Build history of the part. All positions in model axes, mm. A direction names the side the tool comes from. Give positions to 0.01 mm unless a question says otherwise; leave off trailing zeros. Loops run counter-clockwise (first coordinate to the right, second up) from the corner with the lowest first, then second, coordinate; pieces in that order, holes last. Notation, with made-up numbers: (-17, -27) -> (17, -27) arc R13 cw to (17, -4) -> close; hole circle Ø6 at (17, 84.25). An arc over 180 degrees is marked (long way). Answer as a JSON object with one key per item and string values. Group by question number.
Q1. Band-saw the part on C-C, the plane z = 1.5. Count the separate pieces of the cut face and the enclosed holes in it, plus the area to 3 significant figures.
Q2. Band-saw the part on A-A, the plane z = 11.25. Write the cut outline in (x, y).
Q3. Drop flat-ended pins along their axis: pin 1 (1.9 mm diameter, centred on x = 14.58, y = -9.94, fed in from +Z); pin 2 (2.5 mm diameter, centred on x = -15.5, y = 8, fed in from +Z); pin 3 (3.5 mm diameter, centred on x = -16.97, y = -16.97, fed in from -Z). Give the stop position or say it passes through.
Q4. Two-plate mould, pull along Y, no slides. Class faces 4 (the flat face through (15, 10, 2)), 5 (the cylindrical face through (19.797, -19.859, 7.605)), 6 (the flat face through (-21, 0, 7)): pulls with the +Y half, pulls with the -Y half, needs draft (parallel to the pull), parting line crosses it, or undercut.
Q5. Wall check: probe 1 along X at (y, z) = (-0.5, 4.25); probe 2 along X at (y, z) = (14.5, 3); probe 3 along X at (y, z) = (-5.5, 2.5). Give the ranges that are in metal, low to high. Write a range as from..to.
Q6. Band-saw the part on B-B, the plane y = 5. Write the cut outline in (x, z).
Q7. Tool access for faces 1 (the cylindrical face through (-19.02, -16.32, 2.96)), 2 (the flat face through (-4, -17, 2)), 3 (the flat face through (20, -1.1, 14)): list every direction of +Z, -Z, +X, -X, +Y, -Y with a clear straight run to the whole face (end or side of a thin tool).
from build123d import *

# Parameters (mm, degrees)
SKETCH_1_W               = 42
SKETCH_1_H               = 42
EXTRUDE_1_DEPTH          = 15
FILLET_2_R               = 4
SKETCH_25_R              = 1.15
CUT_EXTRUDE_16_DEPTH     = 16
SKETCH_28_R              = 1.45
CUT_EXTRUDE_17_DEPTH     = 2
SKETCH_29_R              = 2.15
CUT_EXTRUDE_18_DEPTH     = 6
SKETCH_30_R              = 19.2
CUT_EXTRUDE_19_DEPTH     = 16
SKETCH_31_R              = 19.35
SKETCH_31_R_2            = 16
EXTRUDE_2_DEPTH          = 5
SKETCH_32_R              = 1.55
CUT_EXTRUDE_22_DEPTH     = 3
PATTERN_CIRCULAR_1_COUNT = 21
SKETCH_33_R              = 18.75
CUT_EXTRUDE_23_DEPTH     = 1
SKETCH_34_W              = 5
SKETCH_34_H              = 2.2
CUT_EXTRUDE_24_DEPTH     = 1.5


with BuildPart() as part:
    # 草图1 → 凸台-拉伸1 (new body)
    with BuildSketch(Plane.XY):
        Rectangle(SKETCH_1_W, SKETCH_1_H)
    extrude(amount=EXTRUDE_1_DEPTH)

    # 圆角2
    fillet_2_edges = [part.edges().sort_by_distance(p)[0] for p in [
        (21, 21, 7.5),
        (21, -21, 7.5),
        (-21, -21, 7.5),
        (-21, 21, 7.5),
    ]]
    fillet(fillet_2_edges, radius=FILLET_2_R)

    # 草图25 → 切除-拉伸16 (cut, through all)
    with BuildSketch(Plane.XY.offset(15)):
        with Locations((-18, 12)):
            Circle(SKETCH_25_R)
        with Locations((18, 12)):
            Circle(SKETCH_25_R)
        with Locations((18, -12)):
            Circle(SKETCH_25_R)
        with Locations((-18, -12)):
            Circle(SKETCH_25_R)
    extrude(amount=-CUT_EXTRUDE_16_DEPTH, mode=Mode.SUBTRACT)

    # 草图28 → 切除-拉伸17 (cut)
    with BuildSketch(Plane.XY.offset(15)):
        with Locations((-15.5, 15.5)):
            Circle(SKETCH_28_R)
        with Locations((15.5, 15.5)):
            Circle(SKETCH_28_R)
        with Locations((15.5, -15.5)):
            Circle(SKETCH_28_R)
        with Locations((-15.5, -15.5)):
            Circle(SKETCH_28_R)
    extrude(amount=-CUT_EXTRUDE_17_DEPTH, mode=Mode.SUBTRACT)

    # 草图29 → 切除-拉伸18 (cut)
    with BuildSketch(Plane(origin=(0, 0, 0), x_dir=(-1, 0, 0), z_dir=(0, 0, -1))):
        with Locations((-16.970562748, 16.970562748)):
            Circle(SKETCH_29_R)
        with Locations((16.970562748, 16.970562748)):
            Circle(SKETCH_29_R)
        with Locations((16.970562748, -16.970562748)):
            Circle(SKETCH_29_R)
        with Locations((-16.970562748, -16.970562748)):
            Circle(SKETCH_29_R)
    extrude(amount=-CUT_EXTRUDE_18_DEPTH, mode=Mode.SUBTRACT)

    # 草图30 → 切除-拉伸19 (cut, through all)
    with BuildSketch(Plane.XY.offset(15)):
        Circle(SKETCH_30_R)
    extrude(amount=-CUT_EXTRUDE_19_DEPTH, mode=Mode.SUBTRACT)

    # 草图31 → 凸台-拉伸2 (add)
    with BuildSketch(Plane(origin=(0, 0, 0), x_dir=(-1, 0, 0), z_dir=(0, 0, -1))):
        Circle(SKETCH_31_R)
        Circle(SKETCH_31_R_2, mode=Mode.SUBTRACT)
    extrude(amount=-EXTRUDE_2_DEPTH)

    # 草图32 → 切除-拉伸22 (cut)
    with BuildSketch(Plane.XY.offset(5)):
        with Locations((17.65, 0)):
            Circle(SKETCH_32_R)
    cut_extrude_22 = extrude(amount=-CUT_EXTRUDE_22_DEPTH, mode=Mode.SUBTRACT)

    # 阵列(圆周)1: 切除-拉伸22 ×21 about axis
    pattern_circular_1_axis = Axis((0, 0, 0), (0, 0, 1))
    for i in range(1, PATTERN_CIRCULAR_1_COUNT):
        add(cut_extrude_22.rotate(pattern_circular_1_axis, i * 360 / PATTERN_CIRCULAR_1_COUNT), mode=Mode.SUBTRACT)

    # 草图33 → 切除-拉伸23 (cut)
    with BuildSketch(Plane(origin=(0, 0, 0), x_dir=(-1, 0, 0), z_dir=(0, 0, -1))):
        Circle(SKETCH_33_R)
    extrude(amount=-CUT_EXTRUDE_23_DEPTH, mode=Mode.SUBTRACT)

    # 草图34 → 切除-拉伸24 (cut)
    with BuildSketch(Plane.XY.offset(15)):
        with Locations((20.745401418, 0)):
            Rectangle(SKETCH_34_W, SKETCH_34_H)
    extrude(amount=-CUT_EXTRUDE_24_DEPTH, mode=Mode.SUBTRACT)


solid = part.part
Worked answers:
{
 "1": {"separate pieces": "1", "enclosed holes": "9", "area": "871 mm2"},
 "2": {"outline": "(-21, -17) arc R4 ccw to (-17, -21) -> (17, -21) arc R4 ccw to (21, -17) -> (21, 17) arc R4 ccw to (17, 21) -> (-17, 21) arc R4 ccw to (-21, 17) -> close; hole circle Ø38.4 at (0, 0); hole circle Ø2.3 at (-18, -12); hole circle Ø2.3 at (-18, 12); hole circle Ø2.3 at (18, -12); hole circle Ø2.3 at (18, 12)"},
 "3": {"pin 1": "z = 2", "pin 2": "z = 5", "pin 3": "z = 6"},
 "4": {"face 4": "undercut", "face 5": "pulls with the -Y half", "face 6": "needs draft"},
 "5": {"probe 1": "-21..-15.99, 15.99..16.18, 19.12..21", "probe 2": "-21..-10.16, -7.49..-6.76, 6.76..9.62, 12.39..21", "probe 3": "-21..-15.02, 15.02..15.34, 18.39..21"},
 "6": {"outline": "(-21, 0) -> (-18.07, 0) -> (-18.07, 1) -> (-15.2, 1) -> (-15.2, 5) -> (-18.54, 5) -> (-18.54, 15) -> (-21, 15) -> close; (15.2, 1) -> (18.07, 1) -> (18.07, 0) -> (21, 0) -> (21, 15) -> (18.54, 15) -> (18.54, 5) -> (18.4, 5) -> (18.4, 2) -> (15.33, 2) -> (15.33, 5) -> (15.2, 5) -> close"},
 "7": {"face 1": "-Z", "face 2": "+Z", "face 3": "+Z, +X"}
}
